```python
from build123d import *

# Parameters (mm, degrees)
IZIM1_W                     = 30
IZIM1_H                     = 30
Y_KSEKLIK_EKSTR_ZYON1_DEPTH = 8
IZIM2_R                     = 12.5
Y_KSEKLIK_EKSTR_ZYON2_DEPTH = 8
IZIM3_R                     = 5.5
KES_EKSTR_ZYON1_DEPTH       = 8
IZIM4_R                     = 1.5
KES_EKSTR_ZYON2_DEPTH       = 8
IZIM5_R                     = 12.5
Y_KSEKLIK_EKSTR_ZYON3_DEPTH = 10
KES_EKSTR_ZYON3_DEPTH       = 10


with BuildPart() as part:
    # Çizim1 → Yükseklik-Ekstrüzyon1 (new body)
    with BuildSketch(Plane.XY):
        with Locations((15, 15)):
            Rectangle(IZIM1_W, IZIM1_H)
    extrude(amount=Y_KSEKLIK_EKSTR_ZYON1_DEPTH)

    # Çizim2 → Yükseklik-Ekstrüzyon2 (add)
    with BuildSketch(Plane.XY.offset(8)):
        with Locations(Location((15, 15, 0), (0, 0, 180))):
            Circle(IZIM2_R)
        Polygon((15, 22.505553499), (8.5, 18.75277675), (8.5, 11.24722325), (15, 7.494446501), (21.5, 11.24722325), (21.5, 18.75277675), align=None, mode=Mode.SUBTRACT)
    extrude(amount=Y_KSEKLIK_EKSTR_ZYON2_DEPTH)

    # Çizim3 → Kes-Ekstrüzyon1 (cut)
    with BuildSketch(Plane.XY.offset(8)):
        with Locations((15, 15)):
            Circle(IZIM3_R)
    extrude(amount=-KES_EKSTR_ZYON1_DEPTH, mode=Mode.SUBTRACT)

    # Çizim4 → Kes-Ekstrüzyon2 (cut)
    with BuildSketch(Plane.XY.offset(8)):
        with Locations((3.5, 26.5)):
            Circle(IZIM4_R)
        with Locations((26.5, 26.5)):
            Circle(IZIM4_R)
        with Locations((26.5, 3.5)):
            Circle(IZIM4_R)
        with Locations((3.5, 3.5)):
            Circle(IZIM4_R)
    extrude(amount=-KES_EKSTR_ZYON2_DEPTH, mode=Mode.SUBTRACT)

    # Çizim5 → Yükseklik-Ekstrüzyon3 (add)
    with BuildSketch(Plane.XY.offset(16)):
        with Locations(Location((15, 15, 0), (0, 0, 180))):
            Circle(IZIM5_R)
        Polygon((15, 22.505553499), (8.5, 18.75277675), (8.5, 11.24722325), (15, 7.494446501), (21.5, 11.24722325), (21.5, 18.75277675), align=None, mode=Mode.SUBTRACT)
    extrude(amount=Y_KSEKLIK_EKSTR_ZYON3_DEPTH)

    # Çizim6 → Kes-Ekstrüzyon3 (cut)
    with BuildSketch(Plane.XY.offset(8)):
        with BuildLine():
            Line((10, 30), (30, 30))
            Line((30, 30), (30, 10))
            ThreePointArc((30, 10), (23.838834765, 23.838834765), (10, 30))
        make_face()
    extrude(amount=-KES_EKSTR_ZYON3_DEPTH, mode=Mode.SUBTRACT)


solid = part.part
```
CAD build for the part. Positions are in the model's coordinates, mm. A direction names the side the tool comes from. Give positions to 0.01 mm unless a question says otherwise; leave off trailing zeros. Loops run counter-clockwise (first coordinate to the right, second up) from the corner with the lowest first, then second, coordinate; pieces in that order, holes last. Notation, with made-up numbers: (4.5, -2) -> (61.5, -2) arc R36 ccw to (61.5, 35) -> close; hole circle Ø10 at (49, 45). An arc over 180 degrees is marked (long way). Use a Markdown table: item, result.
1. Wall check: L1, parallel to Y at x = 3.5, z = 3; L2, parallel to Z at x = 4.75, y = 4.75; L3, parallel to X at y = 20, z = 3. Give the ranges that are in metal, low to high. Write a range as [from, to].
Check result:
| item | result |
|---|---|
| L1 | y = [0, 2], [5, 25], [28, 30] |
| L2 | z = [0, 8] |
| L3 | x = [0, 12.71], [17.29, 26.88] |
2. Slice it at D-D (z = 8.75). List the corners of the cut face in (x, y), plus the area to 3 significant figures.
Check result:
| item | result |
|---|---|
| outline | circle Ø25 at (15, 15); hole (8.5, 11.25) -> (15, 7.49) -> (21.5, 11.25) -> (21.5, 18.75) -> (15, 22.51) -> (8.5, 18.75) -> close |
| area | 345 mm^2 |
3. Which spindle directions (+Z, -Z, +X, -X, +Y, -Y) get a long thin tool onto all of the face, cutting with end or side? Do faces 4 (the flat face through (18.2, 9.34, 16.87)), 5 (the cylindrical face through (25, 3.57, 4.06)). Say none if no direction does.
Check result:
| item | result |
|---|---|
| face 4 | +Z |
| face 5 | +Z, -Z |
4. Slice it at B-B (x = 3.5). List the corners of the cut face in (y, z), plus the area to 3 significant figures.
Check result:
| item | result |
|---|---|
| outline | (0, 0) -> (2, 0) -> (2, 8) -> (0, 8) -> close; (5, 0) -> (25, 0) -> (25, 8) -> (19.9, 8) -> (19.9, 26) -> (10.1, 26) -> (10.1, 8) -> (5, 8) -> close; (28, 0) -> (30, 0) -> (30, 8) -> (28, 8) -> close |
| area | 368 mm^2 |
5. Mould opens along X. For faces 1 (the cylindrical face through (3.305, 27.987, 4.056)), 2 (the cylindrical face through (23.991, 23.685, 4.056)), 3 (the flat face through (8, 15, 0)) say: pulls with the +X half, pulls with the -X half, needs draft (parallel to the pull), parting line crosses it, or undercut.
Check result:
| item | result |
|---|---|
| face 1 | undercut |
| face 2 | pulls with the +X half |
| face 3 | needs draft |
6. Slice it at C-C (y = 15). List the corners of the cut face in (x, z).
Check result:
| item | result |
|---|---|
| outline | (0, 0) -> (9.5, 0) -> (9.5, 8) -> (8.5, 8) -> (8.5, 26) -> (2.5, 26) -> (2.5, 8) -> (0, 8) -> close; (20.5, 0) -> (29.13, 0) -> (29.13, 8) -> (27.5, 8) -> (27.5, 26) -> (21.5, 26) -> (21.5, 8) -> (20.5, 8) -> close |
7. Flat gauge pins, fed straight in: pin 1 (4 mm diameter, centred on y = 15, z = 16.5, fed in from +X); pin 2 (4 mm diameter, centred on x = 12, z = 9, fed in from +Y); pin 3 (2 mm diameter, centred on x = 12.5, z = 23.5, fed in from -Y); pin 4 (1.8 mm diameter, centred on x = 3.5, y = 3.5, fed in from +Z). Where does each tip first touch, or does it go through?
Check result:
| item | result |
|---|---|
| pin 1 | stops at x = 27.5 |
| pin 2 | stops at y = 29.98 |
| pin 3 | stops at y = 2.59 |
| pin 4 | passes through |
8. Slice it at A-A (z = 5). List the corners of the cut face in (x, y), plus the area to 3 significant figures.
Check result:
| item | result |
|---|---|
| outline | (0, 0) -> (30, 0) -> (30, 10) arc R21.13 ccw to (10, 30) -> (0, 30) -> close; hole circle Ø3 at (3.5, 3.5); hole circle Ø3 at (3.5, 26.5); hole circle Ø11 at (15, 15); hole circle Ø3 at (26.5, 3.5) |
| area | 689 mm^2 |
